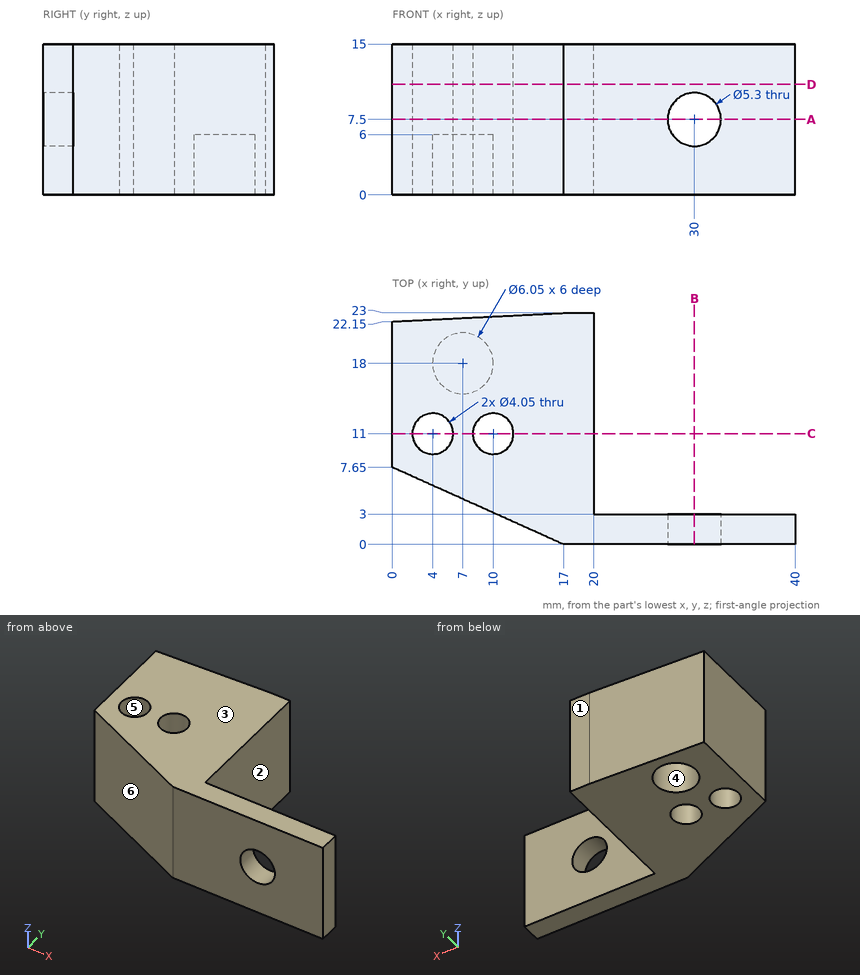
Can you work these out from the drawing? Everything is in mm from the part's minimum corner. A direction names the side the tool comes from. Coordinates: 2 decimals unless noted, no trailing zeros. Write each loop counter-clockwise with the first axis right and the second up, starting at its lowest first coordinate (ties: lowest second). Pieces come first, ordered by that corner, then holes. Notation, with made-up numbers: (11.25, -39) - (22.25, -39) arc R21 ccw to (22.25, -34) - close; hole circle Ø4 at (85, 9). An arc over 180 degrees is marked (long way). Use a Markdown table: item, result.
Q1. I'm going to push flat-ended pins straight in: pin 1 Ø4 at (y, z) = (7.5, 11.5) entering from +X; pin 2 Ø3.5 at (x, y) = (7, 18) entering from -Z; pin 3 Ø5 at (x, z) = (7, 4.5) entering from +Y (3 decimals). Where does each tip first touch, or does it pass through?
Geometry check:
| item | result |
|---|---|
| pin 1 | stops at x = 20 |
| pin 2 | stops at z = 6 |
| pin 3 | stops at y = 22.625 |
Q2. Thinking about a two-plate mould opening in Y: for the marked faces 3, 4, 5 and 6, which applies, +Y half, -Y half, draft (parallel to the pull), parting line (faces both ways), or undercut?
Geometry check:
| item | result |
|---|---|
| face 3 | draft |
| face 4 | undercut |
| face 5 | undercut |
| face 6 | -Y half |
Q3. Please list where these lines run through material, in increasing order: L1, parallel to Z at x = 30, y = 0.95; L2, parallel to Y at x = 37, z = 2.75; L3, parallel to X at y = 16, z = 9.5.
Geometry check:
| item | result |
|---|---|
| L1 | z = 0 to 4.85, 10.15 to 15 |
| L2 | y = 0 to 3 |
| L3 | x = 0 to 20 |
Q4. Imagine slicing it at C-C (y = 11). List the corners of the cut face in (x, z) for me (3 decimals).
Geometry check:
| item | result |
|---|---|
| outline | (0, 0) - (1.975, 0) - (1.975, 15) - (0, 15) - close; (6.025, 0) - (7.975, 0) - (7.975, 15) - (6.025, 15) - close; (12.025, 0) - (20, 0) - (20, 15) - (12.025, 15) - close |
Q5. Imagine slicing it at B-B (x = 30). List the corners of the cut face in (y, z) for me.
Geometry check:
| item | result |
|---|---|
| outline | (0, 0) - (3, 0) - (3, 4.85) - (0, 4.85) - close; (0, 10.15) - (3, 10.15) - (3, 15) - (0, 15) - close |
Q6. Imagine slicing it at A-A (z = 7.5). List the corners of the cut face in (x, y) for me (3 decimals).
Geometry check:
| item | result |
|---|---|
| outline | (0, 7.65) - (17, 0) - (27.35, 0) - (27.35, 3) - (20, 3) - (20, 23) - (17, 23) - (0, 22.15) - close; (32.65, 0) - (40, 0) - (40, 3) - (32.65, 3) - close; hole circle Ø4.05 at (4, 11); hole circle Ø4.05 at (10, 11) |
Q7. Which directions (+Z, -Z, +X, -X, +Y, -Y) give clear straight access to the entire face, cutting with the end or side of a thin tool? Please do the marked faces 1 and 2.
Geometry check:
| item | result |
|---|---|
| face 1 | +Z, -Z, +X, -X, +Y |
| face 2 | +Z, -Z, +X, +Y |
Q8. Imagine slicing it at D-D (z = 11). List the corners of the cut face in (x, y) for me (3 decimals).
Geometry check:
| item | result |
|---|---|
| outline | (0, 7.65) - (17, 0) - (40, 0) - (40, 3) - (20, 3) - (20, 23) - (17, 23) - (0, 22.15) - close; hole circle Ø4.05 at (4, 11); hole circle Ø4.05 at (10, 11) |
